Read the model definition and answer for the solid it produces. Units are mm, in the model's axes. Face numbers are marked on the shaded views. Coordinates: 2 decimals unless noted, no trailing zeros. Write each loop counter-clockwise with the first axis right and the second up, starting at its lowest first coordinate (ties: lowest second). Pieces come first, ordered by that corner, then holes.
1) Each of these flat-tipped pins is pushed along its axis until it touches: pin 1 Ø1.5 at (x, z) = (34, 1.5) entering from +Y; pin 2 Ø1.4 at (y, z) = (9, 1.5) entering from -X; pin 3 Ø0.6 at (x, z) = (25, 1) entering from -Y; pin 4 Ø1 at (x, y) = (37.5, 39.5) entering from -Z. Where does it stop, or does it pass through?
2) The part is cut by section A-A (x = 2.5). Determine the outline of the cut face in (y, z).
3) The part is cut by section B-B (y = 2.5). Determine the outline of the cut face in (x, z), then the cut area to 3 significant figures.
4) Determine the mould class of the marked faces 1 and 2 for opening direction Y: +Y half, -Y half, draft (parallel to the pull), parting line (faces both ways), or undercut.
5) The part is cut by section D-D (y = 15). Determine the outline of the cut face in (x, z), then the cut area to 3 significant figures.
6) The part is cut by section C-C (x = 37.5). Determine the outline of the cut face in (y, z), then the cut area to 3 significant figures.
7) Find the intervals of material crossed by line 1 (Y direction, x = 37.5, z = 2.15); line 2 (X direction, y = 39.5, z = 3.1); line 3 (Y direction, x = 37.5, z = 2.8), in increasing order.
from build123d import *

# Parameters (mm, degrees)
CYLINDER016_R     = 0.8
CYLINDER016_DEPTH = 20
CYLINDER017_R     = 0.8
CYLINDER017_DEPTH = 20
CYLINDER018_R     = 0.8
CYLINDER018_DEPTH = 20
CYLINDER019_R     = 0.8
CYLINDER019_DEPTH = 20
BOX010_W          = 39.8
BOX010_H          = 1
BOX010_DEPTH      = 0.8
BOX009_W          = 39.8
BOX009_H          = 1
BOX009_DEPTH      = 0.8
BOX007_W          = 20
BOX007_H          = 7.2
BOX007_DEPTH      = 10
BOX006_W          = 42
BOX006_H          = 44
BOX006_DEPTH      = 1
BOX005_W          = 39.8
BOX005_H          = 41.8
BOX005_DEPTH      = 1


with BuildPart() as zylinder016:
    # Cylinder016 → Cylinder016 (new body)
    with BuildSketch(Plane(origin=(37.5, 2.5, -10), x_dir=(1, 0, 0), z_dir=(0, 0, 1))):
        Circle(CYLINDER016_R)
    extrude(amount=CYLINDER016_DEPTH)


with BuildPart() as zylinder017:
    # Cylinder017 → Cylinder017 (new body)
    with BuildSketch(Plane(origin=(2.5, 2.5, -10), x_dir=(1, 0, 0), z_dir=(0, 0, 1))):
        Circle(CYLINDER017_R)
    extrude(amount=CYLINDER017_DEPTH)


with BuildPart() as zylinder018:
    # Cylinder018 → Cylinder018 (new body)
    with BuildSketch(Plane(origin=(37.5, 39.5, -10), x_dir=(1, 0, 0), z_dir=(0, 0, 1))):
        Circle(CYLINDER018_R)
    extrude(amount=CYLINDER018_DEPTH)


with BuildPart() as compound006:
    # Cylinder019 → Cylinder019 (new body)
    with BuildSketch(Plane(origin=(2.5, 39.5, -10), x_dir=(1, 0, 0), z_dir=(0, 0, 1))):
        Circle(CYLINDER019_R)
    extrude(amount=CYLINDER019_DEPTH)

    # Compound006: union Zylinder016, Zylinder017, Zylinder018
    add(zylinder016.part)
    add(zylinder017.part)
    add(zylinder018.part)


with BuildPart() as obj1:
    # Box010 → Box010 (new body)
    with BuildSketch(Plane(origin=(0.1, 0.1, 0.7), x_dir=(1, 0, 0), z_dir=(0, 0, 1))):
        with Locations((19.9, 0.5)):
            Rectangle(BOX010_W, BOX010_H)
    extrude(amount=BOX010_DEPTH)


with BuildPart() as compound003:
    # Box009 → Box009 (new body)
    with BuildSketch(Plane(origin=(0.1, 40.9, 0.7), x_dir=(1, 0, 0), z_dir=(0, 0, 1))):
        with Locations((19.9, 0.5)):
            Rectangle(BOX009_W, BOX009_H)
    extrude(amount=BOX009_DEPTH)

    # Compound003: union obj1
    add(obj1.part)


with BuildPart() as obj2:
    # Box007 → Box007 (new body)
    with BuildSketch(Plane(origin=(-12.4, 17.4, 0), x_dir=(1, 0, 0), z_dir=(0, 0, 1))):
        with Locations((10, 3.6)):
            Rectangle(BOX007_W, BOX007_H)
    extrude(amount=BOX007_DEPTH)


with BuildPart() as obj3:
    # Box006 → Box006 (new body)
    with BuildSketch(Plane(origin=(-1, -1, 2.5), x_dir=(1, 0, 0), z_dir=(0, 0, 1))):
        with Locations((21, 22)):
            Rectangle(BOX006_W, BOX006_H)
    extrude(amount=BOX006_DEPTH)


with BuildPart() as lowerpart:
    # Box005 → Box005 (new body)
    with BuildSketch(Plane(origin=(0.1, 0.1, 1.5), x_dir=(1, 0, 0), z_dir=(0, 0, 1))):
        with Locations((19.9, 20.9)):
            Rectangle(BOX005_W, BOX005_H)
    extrude(amount=BOX005_DEPTH)

    # Fusion001: union obj3
    add(obj3.part)

    # Cut003: cut obj2
    add(obj2.part, mode=Mode.SUBTRACT)

    # Fusion003: union Compound003
    add(compound003.part)

    # Cut008: cut Compound006
    add(compound006.part, mode=Mode.SUBTRACT)


solid = lowerpart.part
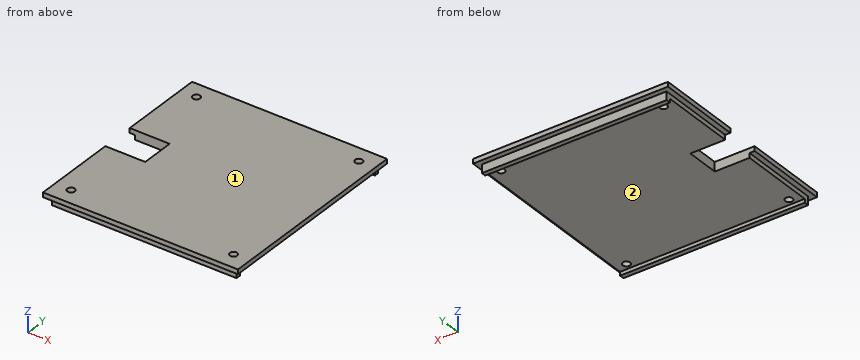
Reported:
1. pin 1: stops at y = 41.9
1. pin 2: stops at x = 0.1
1. pin 3: stops at y = 0.1
1. pin 4: passes through
2. outline: (-1, 2.5) - (0.1, 2.5) - (0.1, 0.7) - (1.1, 0.7) - (1.1, 1.5) - (1.7, 1.5) - (1.7, 3.5) - (-1, 3.5) - close; (3.3, 1.5) - (17.4, 1.5) - (17.4, 3.5) - (3.3, 3.5) - close; (24.6, 1.5) - (38.7, 1.5) - (38.7, 3.5) - (24.6, 3.5) - close; (40.3, 1.5) - (40.9, 1.5) - (40.9, 0.7) - (41.9, 0.7) - (41.9, 2.5) - (43, 2.5) - (43, 3.5) - (40.3, 3.5) - close
3. outline: (-1, 2.5) - (0.1, 2.5) - (0.1, 1.5) - (1.7, 1.5) - (1.7, 3.5) - (-1, 3.5) - close; (3.3, 1.5) - (36.7, 1.5) - (36.7, 3.5) - (3.3, 3.5) - close; (38.3, 1.5) - (39.9, 1.5) - (39.9, 2.5) - (41, 2.5) - (41, 3.5) - (38.3, 3.5) - close
3. area: 75.4 mm2
4. face 1: draft
4. face 2: undercut
5. outline: (-1, 2.5) - (0.1, 2.5) - (0.1, 1.5) - (39.9, 1.5) - (39.9, 2.5) - (41, 2.5) - (41, 3.5) - (-1, 3.5) - close
5. area: 81.8 mm2
6. outline: (-1, 2.5) - (0.1, 2.5) - (0.1, 0.7) - (1.1, 0.7) - (1.1, 1.5) - (1.7, 1.5) - (1.7, 3.5) - (-1, 3.5) - close; (3.3, 1.5) - (38.7, 1.5) - (38.7, 3.5) - (3.3, 3.5) - close; (40.3, 1.5) - (40.9, 1.5) - (40.9, 0.7) - (41.9, 0.7) - (41.9, 2.5) - (43, 2.5) - (43, 3.5) - (40.3, 3.5) - close
6. area: 81.0 mm2
7. line 1: y = 0.1 to 1.7, 3.3 to 38.7, 40.3 to 41.9
7. line 2: x = -1 to 1.7, 3.3 to 36.7, 38.3 to 41
7. line 3: y = -1 to 1.7, 3.3 to 38.7, 40.3 to 43
